Build history of the part. All positions in model axes, mm. Face numbers are marked on the shaded views. A direction names the side the tool comes from. Give positions to 0.01 mm unless a question says otherwise; leave off trailing zeros. Write each loop counter-clockwise with the first axis right and the second up, starting at its lowest first coordinate (ties: lowest second). Pieces come first, ordered by that corner, then holes. Notation, with made-up numbers: (20, 77) -> (44, 77) arc R17 cw to (44, 83) -> close; hole circle Ø5 at (6, -5.5). An arc over 180 degrees is marked (long way). Put each result on its own line as item: value.
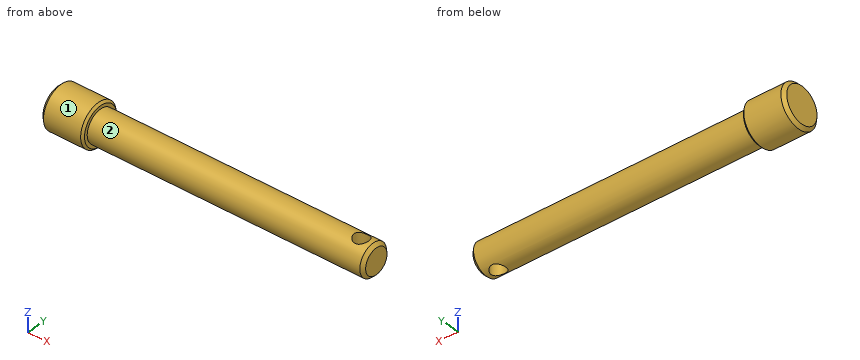
from build123d import *

# Parameters (mm, degrees)
CHANFREIN1_SIZE         = 3
CHANFREIN2_SIZE         = 3
ESQUISSE2_R             = 7
ENL_V_MAT_EXTRU_1_DEPTH = 45
CHANFREIN3_SIZE         = 2


with BuildPart() as part:
    # Esquisse1 → Révolution1 (revolve)
    with BuildSketch(Plane.XY, mode=Mode.PRIVATE) as r_volution1_sk:
        Polygon((0, 0), (0, 20), (40, 20), (40, 15), (300, 15), (300, 0), align=None)
    revolve(r_volution1_sk.sketch.rotate(Axis((0, 0, 0), (1, 0, 0)), 90), axis=Axis((0, 0, 0), (1, 0, 0)))

    # Chanfrein1
    chanfrein1_edges = [part.edges().sort_by_distance(p)[0] for p in [
        (0, 0, -20),
    ]]
    chamfer(chanfrein1_edges, length=CHANFREIN1_SIZE)

    # Chanfrein2
    chanfrein2_edges = [part.edges().sort_by_distance(p)[0] for p in [
        (300, 0, -15),
    ]]
    chamfer(chanfrein2_edges, length=CHANFREIN2_SIZE)

    # Esquisse2 → Enlèv. mat.-Extru.1 (cut, symmetric)
    with BuildSketch(Plane.XY):
        with Locations((286, 0)):
            Circle(ESQUISSE2_R)
    extrude(amount=ENL_V_MAT_EXTRU_1_DEPTH, both=True, mode=Mode.SUBTRACT)

    # Chanfrein3
    chanfrein3_edges = [part.edges().sort_by_distance(p)[0] for p in [
        (40, 0, -20),
    ]]
    chamfer(chanfrein3_edges, length=CHANFREIN3_SIZE)


solid = part.part
1) Slice it at D-D (x = 145.5). Write the cut outline in (y, z), plus the area to 3 significant figures.
Filled sheet:
outline: circle Ø30 at (0, 0)
area: 707 mm2
2) Pin check, flat tips, straight feed: pin 1 (11 mm diameter, centred on x = 286, y = 0, fed in from +Z); pin 2 (12 mm diameter, centred on x = 157.5, z = -14.5, fed in from -Y); pin 3 (1.5 mm diameter, centred on x = 145, y = -1.5, fed in from -Z); pin 4 (1.5 mm diameter, centred on x = 194, z = 13, fed in from +Y). Stop position of each tip, or through.
Filled sheet:
pin 1: through
pin 2: y = -12.36
pin 3: z = -14.98
pin 4: y = 8.66
3) Wall check: L1, parallel to X at y = 0, z = -8.5; L2, parallel to Y at x = 286, z = 5; L3, parallel to Y at x = 286, z = -3. Give the ranges that are in metal, low to high.
Filled sheet:
L1: 0 to 279, 293 to 300
L2: -14.14 to -7, 7 to 14.14
L3: -14.7 to -7, 7 to 14.7
4) Tool access for the marked faces 1 and 2: list every direction of +Z, -Z, +X, -X, +Y, -Y with a clear straight run to the whole face (end or side of a thin tool).
Filled sheet:
face 1: +X, -X
face 2: +X
5) Slice it at C-C (x = 286). Write the cut outline in (y, z).
Filled sheet:
outline: (-7, -13.27) -> (-7, 13.27) arc R15 ccw to start; (7, -13.27) arc R15 ccw to (7, 13.27) -> close
6) Slice it at A-A (y = 0). Write the cut outline in (x, z), plus the area to 3 significant figures.
Filled sheet:
outline: (0, -17) -> (3, -20) -> (38, -20) -> (40, -18) -> (40, -15) -> (279, -15) -> (279, 15) -> (40, 15) -> (40, 18) -> (38, 20) -> (3, 20) -> (0, 17) -> close; (293, -15) -> (297, -15) -> (300, -12) -> (300, 12) -> (297, 15) -> (293, 15) -> close
area: 8,960 mm2
7) Slice it at B-B (z = 0). Write the cut outline in (x, y), plus the area to 3 significant figures.
Filled sheet:
outline: (0, -17) -> (3, -20) -> (38, -20) -> (40, -18) -> (40, -15) -> (297, -15) -> (300, -12) -> (300, 12) -> (297, 15) -> (40, 15) -> (40, 18) -> (38, 20) -> (3, 20) -> (0, 17) -> close; hole circle Ø14 at (286, 0)
area: 9,220 mm2
